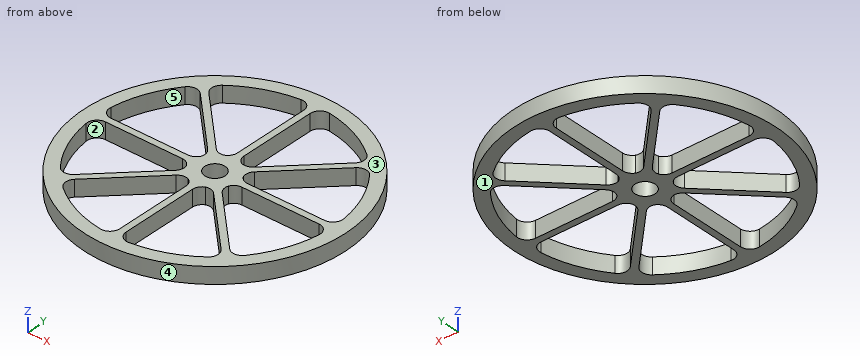
```python
from build123d import *

# Parameters (mm, degrees)
MODEL_R         = 40
MODEL_R_2       = 3.1
EXTRUDE_1_DEPTH = 5


with BuildPart() as part:
    # Model → 凸台-拉伸1 (new body)
    with BuildSketch(Plane.XY):
        with Locations((58.671935635, 46.97216953)):
            Circle(MODEL_R)
        with Locations((58.671935635, 46.97216953)):
            Circle(MODEL_R_2, mode=Mode.SUBTRACT)
        with BuildLine():
            Line((57.671935635, 56.13732092), (57.671935635, 79.728848239))
            ThreePointArc((57.671935635, 79.728848239), (56.66053953, 81.975057166), (54.308299271, 82.706728121))
            ThreePointArc((54.308299271, 82.706728121), (44.895332069, 80.231832701), (36.489343796, 75.325875096))
            ThreePointArc((36.489343796, 75.325875096), (35.343428251, 73.145220564), (36.216572772, 70.841745955))
            Line((36.216572772, 70.841745955), (52.898301717, 54.16001701))
            ThreePointArc((52.898301717, 54.16001701), (54.342318321, 53.358794002), (55.991568665, 53.443147825))
            ThreePointArc((55.991568665, 53.443147825), (57.217411925, 54.549696766), (57.671935635, 56.13732092))
        make_face(mode=Mode.SUBTRACT)
        with BuildLine():
            Line((64.445569552, 54.16001701), (81.127298497, 70.841745955))
            ThreePointArc((81.127298497, 70.841745955), (82.000443018, 73.145220564), (80.854527474, 75.325875096))
            ThreePointArc((80.854527474, 75.325875096), (72.4485392, 80.231832701), (63.035571998, 82.706728121))
            ThreePointArc((63.035571998, 82.706728121), (60.683331739, 81.975057166), (59.671935635, 79.728848239))
            Line((59.671935635, 79.728848239), (59.671935635, 56.13732092))
            ThreePointArc((59.671935635, 56.13732092), (60.126459344, 54.549696766), (61.352302605, 53.443147825))
            ThreePointArc((61.352302605, 53.443147825), (63.001552948, 53.358794002), (64.445569552, 54.16001701))
        make_face(mode=Mode.SUBTRACT)
        with BuildLine():
            Line((67.837087024, 47.97216953), (91.428614343, 47.97216953))
            ThreePointArc((91.428614343, 47.97216953), (93.67482327, 48.983565635), (94.406494225, 51.335805894))
            ThreePointArc((94.406494225, 51.335805894), (91.931598805, 60.748773096), (87.0256412, 69.154761369))
            ThreePointArc((87.0256412, 69.154761369), (84.844986668, 70.300676914), (82.54151206, 69.427532393))
            Line((82.54151206, 69.427532393), (65.859783114, 52.745803448))
            ThreePointArc((65.859783114, 52.745803448), (65.058560106, 51.301786844), (65.142913929, 49.652536502))
            ThreePointArc((65.142913929, 49.652536502), (66.24946287, 48.42669324), (67.837087024, 47.97216953))
        make_face(mode=Mode.SUBTRACT)
        with BuildLine():
            Line((65.859783114, 41.198535613), (82.54151206, 24.516806668))
            ThreePointArc((82.54151206, 24.516806668), (84.844986668, 23.643662147), (87.0256412, 24.789577691))
            ThreePointArc((87.0256412, 24.789577691), (91.931598805, 33.195565965), (94.406494225, 42.608533167))
            ThreePointArc((94.406494225, 42.608533167), (93.67482327, 44.960773426), (91.428614343, 45.97216953))
            Line((91.428614343, 45.97216953), (67.837087024, 45.97216953))
            ThreePointArc((67.837087024, 45.97216953), (66.24946287, 45.51764582), (65.142913929, 44.291802559))
            ThreePointArc((65.142913929, 44.291802559), (65.058560106, 42.642552216), (65.859783114, 41.198535613))
        make_face(mode=Mode.SUBTRACT)
        with BuildLine():
            Line((59.671935635, 37.807018141), (59.671935635, 14.215490822))
            ThreePointArc((59.671935635, 14.215490822), (60.683331739, 11.969281895), (63.035571998, 11.23761094))
            ThreePointArc((63.035571998, 11.23761094), (72.4485392, 13.71250636), (80.854527474, 18.618463965))
            ThreePointArc((80.854527474, 18.618463965), (82.000443018, 20.799118497), (81.127298497, 23.102593105))
            Line((81.127298497, 23.102593105), (64.445569552, 39.784322051))
            ThreePointArc((64.445569552, 39.784322051), (63.001552948, 40.585545059), (61.352302606, 40.501191236))
            ThreePointArc((61.352302606, 40.501191236), (60.126459344, 39.394642295), (59.671935635, 37.807018141))
        make_face(mode=Mode.SUBTRACT)
        with BuildLine():
            Line((52.898301717, 39.784322051), (36.216572772, 23.102593105))
            ThreePointArc((36.216572772, 23.102593105), (35.343428251, 20.799118497), (36.489343796, 18.618463965))
            ThreePointArc((36.489343796, 18.618463965), (44.895332069, 13.71250636), (54.308299271, 11.23761094))
            ThreePointArc((54.308299271, 11.23761094), (56.66053953, 11.969281895), (57.671935635, 14.215490822))
            Line((57.671935635, 14.215490822), (57.671935635, 37.807018141))
            ThreePointArc((57.671935635, 37.807018141), (57.217411925, 39.394642295), (55.991568664, 40.501191236))
            ThreePointArc((55.991568664, 40.501191236), (54.342318321, 40.585545059), (52.898301717, 39.784322051))
        make_face(mode=Mode.SUBTRACT)
        with BuildLine():
            Line((49.506784245, 45.97216953), (25.915256926, 45.97216953))
            ThreePointArc((25.915256926, 45.97216953), (23.669047999, 44.960773426), (22.937377044, 42.608533167))
            ThreePointArc((22.937377044, 42.608533167), (25.412272464, 33.195565965), (30.318230069, 24.789577691))
            ThreePointArc((30.318230069, 24.789577691), (32.498884601, 23.643662147), (34.80235921, 24.516806668))
            Line((34.80235921, 24.516806668), (51.484088155, 41.198535613))
            ThreePointArc((51.484088155, 41.198535613), (52.285311163, 42.642552216), (52.20095734, 44.291802559))
            ThreePointArc((52.20095734, 44.291802559), (51.0944084, 45.51764582), (49.506784245, 45.97216953))
        make_face(mode=Mode.SUBTRACT)
        with BuildLine():
            Line((51.484088155, 52.745803448), (34.80235921, 69.427532393))
            ThreePointArc((34.80235921, 69.427532393), (32.498884601, 70.300676914), (30.318230069, 69.154761369))
            ThreePointArc((30.318230069, 69.154761369), (25.412272464, 60.748773096), (22.937377044, 51.335805894))
            ThreePointArc((22.937377044, 51.335805894), (23.669047999, 48.983565635), (25.915256926, 47.97216953))
            Line((25.915256926, 47.97216953), (49.506784245, 47.97216953))
            ThreePointArc((49.506784245, 47.97216953), (51.094408399, 48.42669324), (52.20095734, 49.652536501))
            ThreePointArc((52.20095734, 49.652536501), (52.285311163, 51.301786844), (51.484088155, 52.745803448))
        make_face(mode=Mode.SUBTRACT)
    extrude(amount=EXTRUDE_1_DEPTH)


solid = part.part
```
Design review of the part built by this model. Coordinates are the model's own, in mm. Face numbers are marked on the shaded views. A direction names the side the tool comes from. Round coordinates to 2 decimals unless told otherwise and drop trailing zeros. Write each loop counter-clockwise with the first axis right and the second up, starting at its lowest first coordinate (ties: lowest second). Pieces come first, ordered by that corner, then holes. Notation, with made-up numbers: (-19, -23) -> (-10, -23) arc R14 ccw to (-10, -3) -> close; hole circle Ø5 at (47.5, 7). An arc over 180 degrees is marked (long way). Write item = value, one per line. Start each with the question number.
1) Take a section at A-A, the plane x = 45.5. State the section outline as (y, z) points.
2) Take a section at B-B, the plane x = 92.5. State the section outline as (y, z) points.
3) Clearance check with flat-ended pins moving along their axes: pin 1 (3 mm diameter, centred on y = 19, z = 4, fed in from +X); pin 2 (2.5 mm diameter, centred on x = 77.5, z = 3, fed in from +Y); pin 3 (6 mm diameter, centred on x = 29.5, y = 52.5, fed in from -Z); pin 4 (1.5 mm diameter, centred on y = 42.5, z = 1.5, fed in from -X). State where each tip first meets the part, or that it passes through.
4) Wall thickness on probe 1 along X at (y, z) = (55, 0.2); probe 2 along Y at (x, z) = (91.5, 3); probe 3 along X at (y, z) = (78, 2.95): over which ranges is each line inside the solid? List them lowest first. Write a range as from..to.
5) Mouldability with a two-part tool opening along X and no side actions: class the marked faces 3, 4 and 5 as +X half, -X half, draft (parallel to the pull), parting line (faces both ways), or undercut.
6) Take a section at C-C, the plane z = 0.75. Count the separate pieces of the cut face and the enclosed holes in it, plus the area to 3 significant figures.
7) Tool access review of the marked faces 1 and 2: name each direction out of +Z, -Z, +X, -X, +Y, -Y from which nothing blocks a thin tool from reaching the whole face with its end or side.
Results list:
q1.outline = (9.2, 0) -> (13.47, 0) -> (13.47, 5) -> (9.2, 5) -> close; (32.39, 0) -> (35.21, 0) -> (35.21, 5) -> (32.39, 5) -> close; (45.97, 0) -> (47.97, 0) -> (47.97, 5) -> (45.97, 5) -> close; (58.73, 0) -> (61.56, 0) -> (61.56, 5) -> (58.73, 5) -> close; (80.48, 0) -> (84.74, 0) -> (84.74, 5) -> (80.48, 5) -> close
q2.outline = (25.63, 0) -> (34.66, 0) -> (34.66, 5) -> (25.63, 5) -> close; (45.77, 0) -> (48.17, 0) -> (48.17, 5) -> (45.77, 5) -> close; (59.29, 0) -> (68.32, 0) -> (68.32, 5) -> (59.29, 5) -> close
q3.pin_1 = 88.66
q3.pin_2 = 82.9
q3.pin_3 = through
q3.pin_4 = 18.85
q4.probe_1 = 19.49..23.58, 49.23..52.06, 57.45..59.9, 65.29..68.11, 93.77..97.86
q4.probe_2 = 24.12..32.2, 45.97..47.97, 61.75..69.83
q4.probe_3 = 33.43..40.42, 57.67..59.67, 76.93..83.92
q5.face_3 = draft
q5.face_4 = parting line
q5.face_5 = undercut
q6.separate_pieces = 1
q6.enclosed_holes = 9
q6.area = 1,590 mm²
q7.face_1 = -Z, +X, -X, +Y, -Y
q7.face_2 = +Z, -Z
